```python
from build123d import *

# Parameters (mm, degrees)
MAINBASESKETCH_W                 = 7.9
MAINBASESKETCH_H                 = 3.2
MAINBASEEXTRUDE_DEPTH            = 7.9
MAINBASESHELL_T                  = -1.2
SLIMYELLOWUNDEREXT_START         = -0.2
SLIMYELLOWUNDEREXT_DEPTH         = 2
SLIMYELLLOWUPPERCIRCLESKETCH_R   = 2.45
SLIMYELLLOWUPPERCIRCLESKETCH_R_2 = 2
SLIMYELLOWUPPERCIRCLE_DEPTH      = 1.6
MOVE_START                       = 3.2
MOVE_FACE2_OUTLINE_W             = 7.9
MOVE_FACE2_OUTLINE_H             = 15.8
MOVE_FACE2_OUTLINE_R             = 2
MOVE_FACE2_DEPTH                 = 27.8
MOVE_START_2                     = 31
MOVE_FACE2_2_OUTLINE_R           = 2.45
MOVE_FACE2_2_OUTLINE_R_2         = 2
MOVE_FACE2_2_DEPTH               = 1.6
FILLET25_R                       = 7.6
FILLET26_R                       = 7.6
CUT_EXTRUDE55_DEPTH              = 35.461282763
CUT_EXTRUDE57_REACH              = 34.748
SKETCH160_R                      = 0.75
BOSS_EXTRUDE20_DEPTH             = 3.5
BOSS_EXTRUDE22_DEPTH             = 1.2
CUT_EXTRUDE58_DEPTH              = 35.461282763
CUT_EXTRUDE59_DEPTH              = 31.506685799
CUT_EXTRUDE61_DEPTH              = 31.506685799
LPATTERN5_COUNT                  = 5
LPATTERN5_PITCH                  = 4
LPATTERN5_COUNT_DIR2             = 3
LPATTERN5_PITCH_DIR2             = 4
CUT_EXTRUDE62_DEPTH              = 31.506685799


# Read off the part's stored shape, not the designer's step: Move Face2
with BuildPart() as part:
    # MainBaseSketch → MainBaseExtrude (new, symmetric)
    with BuildSketch(Plane.XY):
        with Locations((4.631967213, 1.6)):
            Rectangle(MAINBASESKETCH_W, MAINBASESKETCH_H)
    extrude(amount=MAINBASEEXTRUDE_DEPTH, both=True)

    # MainBaseShell
    mainbaseshell_openings = [part.faces().sort_by_distance(p)[0] for p in [
        (4.631967213, 0, 0),
    ]]
    offset(amount=MAINBASESHELL_T, openings=mainbaseshell_openings, kind=Kind.INTERSECTION)

    # SlimYellowUnderExtSketch → SlimYellowUnderExt (add)
    with BuildSketch(Plane.XZ.offset(-2).offset(SLIMYELLOWUNDEREXT_START)):
        Polygon((1.881967213, 1.952811318), (1.881967213, 2.947188682), (2.384104441, 2.947188682), (2.882626102, 2.45), (2.384104441, 1.952811318), align=None)
        Polygon((6.381308324, 2.45), (6.879829986, 2.947188682), (7.381967213, 2.947188682), (7.381967213, 1.952811318), (6.879829986, 1.952811318), align=None)
        Polygon((1.881967213, -1.952811318), (2.384104441, -1.952811318), (2.882626102, -2.45), (2.384104441, -2.947188682), (1.881967213, -2.947188682), align=None)
        Polygon((7.381967213, -1.952811318), (7.381967213, -2.947188682), (6.879829986, -2.947188682), (6.381308324, -2.45), (6.879829986, -1.952811318), align=None)
    extrude(amount=SLIMYELLOWUNDEREXT_DEPTH)

    # SlimYelllowUpperCircleSketch → SlimYellowUpperCircle (add)
    with BuildSketch(Plane(origin=(0, 3.2, 0), x_dir=(1, 0, 0), z_dir=(0, 1, 0))):
        with Locations((4.647335619, 0)):
            Circle(SLIMYELLLOWUPPERCIRCLESKETCH_R)
        with Locations(Location((4.647335619, 0, 0), (0, 0, 270))):
            Circle(SLIMYELLLOWUPPERCIRCLESKETCH_R_2, mode=Mode.SUBTRACT)
    extrude(amount=SLIMYELLOWUPPERCIRCLE_DEPTH)

    # Move Face2 outline → Move Face2 (add)
    with BuildSketch(Plane(origin=(0, 0, 0), x_dir=(1, 0, 0), z_dir=(0, 1, 0)).offset(MOVE_START)):
        with Locations((4.631967213, 0)):
            Rectangle(MOVE_FACE2_OUTLINE_W, MOVE_FACE2_OUTLINE_H)
        with Locations((4.647335619, 0)):
            Circle(MOVE_FACE2_OUTLINE_R, mode=Mode.SUBTRACT)
    extrude(amount=MOVE_FACE2_DEPTH)

    # Move Face2 2 outline → Move Face2 2 (add)
    with BuildSketch(Plane(origin=(0, 0, 0), x_dir=(1, 0, 0), z_dir=(0, 1, 0)).offset(MOVE_START_2)):
        with Locations((4.647335619, 0)):
            Circle(MOVE_FACE2_2_OUTLINE_R)
        with Locations((4.647335619, 0)):
            Circle(MOVE_FACE2_2_OUTLINE_R_2, mode=Mode.SUBTRACT)
    extrude(amount=MOVE_FACE2_2_DEPTH)

    # Fillet25
    # the kernel refuses this fillet: 7.6 mm, written as the material it takes off along each edge
    with BuildSketch(Plane(origin=(0.681967213, 31, 7.9), x_dir=(0, 0, -1), z_dir=(1, 0, 0))) as fillet25_piece_1_section:
        with BuildLine():
            CenterArc((FILLET25_R, -FILLET25_R), FILLET25_R, 90, 90)
            Line((0, -FILLET25_R), (-FILLET25_R * 0.02, -FILLET25_R))
            Line((-FILLET25_R * 0.02, -FILLET25_R), (-FILLET25_R * 0.02, FILLET25_R * 0.02))
            Line((-FILLET25_R * 0.02, FILLET25_R * 0.02), (FILLET25_R, FILLET25_R * 0.02))
            Line((FILLET25_R, FILLET25_R * 0.02), (FILLET25_R, 0))
        make_face()
    fillet25_piece_1 = extrude(amount=7.9, mode=Mode.PRIVATE)
    fillet25_piece_1 = fillet25_piece_1 - Plane(origin=(4.647335619, 29.251763141, 0), x_dir=(1, 0, 0), z_dir=(0, -1, 0)) * Cylinder(2.45, 47, mode=Mode.PRIVATE)
    add(fillet25_piece_1, mode=Mode.SUBTRACT)

    # Fillet26
    # the kernel refuses this fillet: 7.6 mm, written as the material it takes off along each edge
    with BuildSketch(Plane(origin=(27.581967213, 31, -7.9), x_dir=(0, 0, 1), z_dir=(-1, 0, 0))) as fillet26_piece_1_section:
        with BuildLine():
            CenterArc((FILLET26_R, -FILLET26_R), FILLET26_R, 90, 90)
            Line((0, -FILLET26_R), (0, 0))
            Line((0, 0), (FILLET26_R, 0))
        make_face()
    fillet26_piece_1 = extrude(amount=45.9, mode=Mode.PRIVATE)
    fillet26_piece_1 = fillet26_piece_1 - Plane(origin=(4.647335619, 29.29236393, 0), x_dir=(1, 0, 0), z_dir=(0, -1, 0)) * Cylinder(2.45, 123, mode=Mode.PRIVATE)
    add(fillet26_piece_1, mode=Mode.SUBTRACT)

    # Sketch159 → Cut-Extrude55 (cut, through all)
    with BuildSketch(Plane(origin=(8.581967213, 0, 0), x_dir=(0, 0, -1), z_dir=(1, 0, 0))):
        with BuildLine():
            Line((6.7, 3.204620212), (6.7, 23.463811934))
            ThreePointArc((6.7, 23.463811934), (0, 29.737650856), (-6.7, 23.463811934))
            Line((-6.7, 23.463811934), (-6.7, 3.204620212))
            Line((-6.7, 3.204620212), (6.7, 3.204620212))
        make_face()
    extrude(amount=-CUT_EXTRUDE55_DEPTH, mode=Mode.SUBTRACT)

    # Sketch160 → Cut-Extrude57 (cut, up to next)
    with BuildSketch(Plane(origin=(0, 2, 0), x_dir=(-1, 0, 0), z_dir=(0, -1, 0)), mode=Mode.PRIVATE) as cut_extrude57_sk1:
        with Locations(Location((-6.381967213, 0, 0), (0, 0, 180))):
            Circle(SKETCH160_R)
    cut_extrude57_tool1 = extrude(cut_extrude57_sk1.sketch, amount=-CUT_EXTRUDE57_REACH, mode=Mode.PRIVATE) & part.part
    # Sketch160 → Cut-Extrude57 (cut, up to next)
    with BuildSketch(Plane(origin=(0, 2, 0), x_dir=(-1, 0, 0), z_dir=(0, -1, 0)), mode=Mode.PRIVATE) as cut_extrude57_sk2:
        with Locations(Location((-2.881967213, 0, 0), (0, 0, 180))):
            Circle(SKETCH160_R)
    cut_extrude57_tool2 = extrude(cut_extrude57_sk2.sketch, amount=-CUT_EXTRUDE57_REACH, mode=Mode.PRIVATE) & part.part
    add(cut_extrude57_tool1.solids().sort_by_distance((6.381967, 2, 0))[0], mode=Mode.SUBTRACT)
    add(cut_extrude57_tool2.solids().sort_by_distance((2.881967, 2, 0))[0], mode=Mode.SUBTRACT)

    # Sketch161 → Boss-Extrude20 (add, symmetric)
    with BuildSketch(Plane(origin=(4.631967213, 0, 0), x_dir=(0, 0, -1), z_dir=(1, 0, 0))):
        with BuildLine():
            Line((2.455062292, 30.688052313), (2.455062292, 30.469179439))
            Line((2.455062292, 30.469179439), (2.455062292, 29.272723248))
            ThreePointArc((2.455062292, 29.272723248), (0, 29.737650856), (-2.455062292, 29.272723248))
            Line((-2.455062292, 29.272723248), (-2.455062292, 30.526922148))
            Line((-2.455062292, 30.526922148), (-2.455062292, 30.688052313))
            ThreePointArc((-2.455062292, 30.688052313), (0, 31.033009473), (2.455062292, 30.688052313))
        make_face()
    extrude(amount=BOSS_EXTRUDE20_DEPTH, both=True)

    # Sketch163 → Cut-Extrude58 (cut, through all)
    with BuildSketch(Plane.ZY.offset(-0.681967213)):
        with BuildLine():
            Line((-7.9, 23.4), (-7.9, 0))
            Line((-7.9, 0), (7.9, 0))
            Line((7.9, 0), (7.9, 23.4))
            ThreePointArc((7.9, 23.4), (6.393942446, 28.039773701), (2.45, 30.91049266))
            Line((2.45, 30.91049266), (2.514245173, 32.885555996))
            Line((2.514245173, 32.885555996), (-2.45, 32.885555996))
            Line((-2.45, 32.885555996), (-2.45, 30.91049266))
            ThreePointArc((-2.45, 30.91049266), (-6.393942446, 28.039773701), (-7.9, 23.4))
        make_face()
        with BuildLine():
            Line((6.7, 23.463811934), (6.7, 3.204620212))
            Line((6.7, 3.204620212), (-6.7, 3.204620212))
            Line((-6.7, 3.204620212), (-6.7, 23.463811934))
            ThreePointArc((-6.7, 23.463811934), (0, 29.737650856), (6.7, 23.463811934))
        make_face(mode=Mode.SUBTRACT)
    extrude(amount=-CUT_EXTRUDE58_DEPTH, mode=Mode.SUBTRACT)


with BuildPart() as body_2:
    # Sketch162 → Boss-Extrude22 (new body)
    with BuildSketch(Plane.ZY.offset(-0.681967213)):
        with BuildLine():
            Line((-6.7, 3.204620212), (-6.7, 23.463811934))
            ThreePointArc((-6.7, 23.463811934), (0, 29.737650856), (6.7, 23.463811934))
            Line((6.7, 23.463811934), (6.7, 3.204620212))
            Line((6.7, 3.204620212), (-6.7, 3.204620212))
        make_face()
    extrude(amount=BOSS_EXTRUDE22_DEPTH)

    # Sketch164 → Cut-Extrude59 (cut, through all)
    with BuildSketch(Plane.ZY.offset(-0.681967213)):
        Polygon((0, 27.521885921), (-1.241361972, 28.838648646), (1.278746144, 28.898801022), align=None)
    extrude(amount=CUT_EXTRUDE59_DEPTH, mode=Mode.SUBTRACT)

    # Sketch165 → Cut-Extrude61 (cut, through all)
    with BuildSketch(Plane.ZY.offset(-0.681967213)):
        Polygon((-4.405546645, 23.827298552), (-3.03141738, 22.453169286), (-4.405546645, 21.079040021), (-5.779675911, 22.453169286), align=None)
    cut_extrude61 = extrude(amount=CUT_EXTRUDE61_DEPTH, mode=Mode.SUBTRACT)

    # LPattern5: Cut-Extrude61 5 × 3
    with Locations(*[(0, -i * LPATTERN5_PITCH, j * LPATTERN5_PITCH_DIR2) for i in range(LPATTERN5_COUNT) for j in range(LPATTERN5_COUNT_DIR2) if (i, j) != (0, 0)]):
        add(cut_extrude61, mode=Mode.SUBTRACT)

    # Sketch166 → Cut-Extrude62 (cut, through all)
    with BuildSketch(Plane.ZY.offset(-0.681967213)):
        Polygon((-4.494877975, 24.067352963), (-5.720341085, 25.188203369), (-4.494877975, 26.443555824), (-3.311490851, 25.361189552), align=None)
        Polygon((-4.06895482, 26.742449265), (-2.909533146, 25.682002612), (-1.939612427, 26.742449265), (-2.909533146, 27.689276634), align=None)
        Polygon((-2.529653596, 27.908133687), (-1.326607494, 26.742449265), (-0.609263234, 27.908133687), (-1.326607494, 28.730090652), align=None)
        Polygon((-3.311490851, 24.134603988), (-2.225644972, 23.048758109), (-1.053867228, 24.220535852), (-2.225644972, 25.392313595), align=None)
        Polygon((-1.760283975, 25.682002612), (-0.536126237, 24.457844874), (0.311285226, 25.682002612), (-0.781045381, 26.661241207), align=None)
        Polygon((0.640575983, 24.457844874), (1.865804986, 23.232615872), (3.266618207, 24.633429093), (1.865804986, 26.034242315), align=None)
        Polygon((0.170877374, 27.11002176), (1.253190484, 26.027708649), (2.335503595, 27.11002176), (1.253190484, 28.19233487), align=None)
        Polygon((3.001969531, 26.443555824), (4.270065236, 24.825578524), (5.076744937, 26.443555824), (3.675931716, 27.844369045), align=None)
        Polygon((4.270065236, 23.933022483), (5.15432961, 23.048758109), (5.775380406, 24.339596358), (5.15432961, 25.333835704), align=None)
    extrude(amount=CUT_EXTRUDE62_DEPTH, mode=Mode.SUBTRACT)


solid = body_2.part
```
CAD build for the part. Positions are in the model's coordinates, mm. Give positions to 0.01 mm unless a question says otherwise; leave off trailing zeros. Order: outer loops, then holes, each group sorted by start corner. A loop starts at its lowest first (then second) coordinate and runs counter-clockwise, first axis right, second up.
(1) Saw through at B-B, the plane x = 0.45. State how many separate pieces and enclosed holes the cut face has, then the cut area to 3 significant figures.
(2) Mould opens along Z. For faces 1 (the flat face through (0.09, 15.131, 2.898)), 2 (the flat face through (0, 3.205, 0)) say: released by +Z, released by -Z, zero draft, split by the parting line, or undercut.
(3) Saw through at A-A, the plane y = 22. Give the cut face in (x, z), then the cut area to 3 significant figures.
(4) Saw through at C-C, the plane y = 9.5. Give the cut face in (x, z).
(5) Drill centre lines: L1, parallel to Z at x = 0, y = 19.75; L2, parallel to Z at x = 0.3, y = 24.25; L3, parallel to Z at x = -0.3, y = 26.5. Where is each one in solid material? Low to high.
Results found:
1. separate pieces: 1
1. enclosed holes: 25
1. area: 255 mm2
2. face 1: undercut
2. face 2: zero draft
3. outline: (-0.52, -6.7) - (0.68, -6.7) - (0.68, -5.33) - (-0.52, -5.33) - close; (-0.52, -3.48) - (0.68, -3.48) - (0.68, -1.33) - (-0.52, -1.33) - close; (-0.52, 0.52) - (0.68, 0.52) - (0.68, 2.67) - (-0.52, 2.67) - close; (-0.52, 4.52) - (0.68, 4.52) - (0.68, 6.7) - (-0.52, 6.7) - close
3. area: 9.45 mm2
4. outline: (-0.52, -6.7) - (0.68, -6.7) - (0.68, -4.83) - (-0.52, -4.83) - close; (-0.52, -3.98) - (0.68, -3.98) - (0.68, -0.83) - (-0.52, -0.83) - close; (-0.52, 0.02) - (0.68, 0.02) - (0.68, 3.17) - (-0.52, 3.17) - close; (-0.52, 4.02) - (0.68, 4.02) - (0.68, 6.7) - (-0.52, 6.7) - close
5. L1: z = -6.7 to -4.48, -4.33 to -0.48, -0.33 to 3.52, 3.67 to 6.7
5. L2: z = -6.6 to -4.69, -4.33 to -3.21, -1.08 to 0.85, 2.88 to 4.47, 5.73 to 6.6
5. L3: z = -5.74 to -3.8, -2.16 to -0.94, -0.6 to 0.78, 1.73 to 3.03, 5.02 to 5.74
